Autodesk Inventor part; units mm, degrees
ref_plane "YZ Plane" through (0, 0, 0) normal (1, 0, 0) x (0, 1, 0)
ref_plane "XZ Plane" through (0, 0, 0) normal (0, 1, 0) x (-1, 0, 0)
ref_plane "XY Plane" through (0, 0, 0) normal (0, 0, 1) x (1, 0, 0)
sketch "Sketch1" plane through (0, 0, 0) normal (1, 0, 0) x (0, 1, 0)
  line L0 (12, 12.5) -> (-12, 12.5)
  line L1 (-12, 12.5) -> (-12, -12.5)
  line L2 (-12, -12.5) -> (12, -12.5)
  line L3 (12, -12.5) -> (12, 12.5)
  line L4 (12, 12.5) -> (-12, -12.5) construction
  line L5 (-12, 12.5) -> (12, -12.5) construction
  circle A0 centre (10, 10.5) radius 1.05
  line L6 (12, 0) -> (-12, 0) construction
  circle A1 centre (-2.5, 10.5) radius 1.05
  circle A2 centre (10, -10.5) radius 1.05
  circle A3 centre (-2.5, -10.5) radius 1.05
  point P0 (0, 0)
  dimension "d0" = 24
  dimension "d1" = 25
  dimension "d2" = 2.1
  dimension "d3" = 2
  dimension "d4" = 2
  dimension "d5" = 2.1
  dimension "d6" = 12.5
  dimension "d7" = 2
extrude "Extrusion1" add sketch "Sketch1" along normal mid plane 1.5
properties part number "Booard"
Input: part model. Units: mm. Frame: model coordinates. Give positions to 0.01 mm unless a question says otherwise; leave off trailing zeros. Order: outer loops, then holes, each group sorted by start corner. A loop starts at its lowest first (then second) coordinate and runs counter-clockwise, first axis right, second up. Notation, with made-up numbers: M 14.5,4.25 L 42.5,4.25 A37 cw 42.5,41.25 Z; hole C 4,-35 d6. An arc over 180 degrees is marked long. Answer as a JSON object with one key per item and string values.
1. Cut plane B-B, the plane x = 0.3. Output: boundary loops of the cut face in (y, z), and give its area (3 significant figures).
Result sheet:
{"outline": "M -12,-12.5 L 12,-12.5 L 12,12.5 L -12,12.5 Z; hole C -2.5,-10.5 d2.1; hole C -2.5,10.5 d2.1; hole C 10,-10.5 d2.1; hole C 10,10.5 d2.1", "area": "586 mm²"}
2. Cut plane C-C, the plane y = 10. Output: boundary loops of the cut face in (x, z).
Result sheet:
{"outline": "M -0.75,-12.5 L 0.75,-12.5 L 0.75,-11.55 L -0.75,-11.55 Z; M -0.75,-9.45 L 0.75,-9.45 L 0.75,9.45 L -0.75,9.45 Z; M -0.75,11.55 L 0.75,11.55 L 0.75,12.5 L -0.75,12.5 Z"}
3. Ray query, line 1 (Z direction, x = -0.25, y = -2.5); line 2 (Y direction, x = -0.25, z = 10). Return the intervals inside material, ascending. Write a range as [from, to].
Result sheet:
{"line 1": "[-12.5, -11.55], [-9.45, 9.45], [11.55, 12.5]", "line 2": "[-12, -3.42], [-1.58, 9.08], [10.92, 12]"}
4. Pull-direction query (Z, two-part tool) for faces 1 (the flat face through (0.75, 0, 0)), 2 (the flat face through (0, 0, -12.5)), 3 (the cylindrical face through (-0.01, 11, -10.82)); classes: +Z half, -Z half, draft (parallel to the pull), parting line (faces both ways), or undercut.
Result sheet:
{"face 1": "draft", "face 2": "-Z half", "face 3": "undercut"}
5. First-contact query: P1, Ø2.5, axis at y = -2.5, z = -10.5, coming from the -X side. Flat tip, straight axial feed; report the tip coordinate or a pass-through.
Result sheet:
{"P1": "x = -0.75"}
6. Cut plane A-A, the plane z = -10.5. Output: boundary loops of the cut face in (x, y).
Result sheet:
{"outline": "M -0.75,-12 L 0.75,-12 L 0.75,-3.55 L -0.75,-3.55 Z; M -0.75,-1.45 L 0.75,-1.45 L 0.75,8.95 L -0.75,8.95 Z; M -0.75,11.05 L 0.75,11.05 L 0.75,12 L -0.75,12 Z"}
